from build123d import *

# Parameters (mm, degrees)
F1_DEPTH = 50.8
F3_DEPTH = 25.4
F4_W     = 12.7
F4_H     = 20.7277986608
F5_DEPTH = 19.05
F7_DEPTH = 25.4


with BuildPart() as f1:
    # F0 (on Right) → F1 (new body)
    with BuildSketch(Plane.YZ):
        Polygon((0, 0), (0, 31.7254364491), (-12.6999762453, 31.75), (-12.6999762453, 12.7), (-33.4277749062, 12.7), (-33.4277749062, 0), align=None)
    extrude(amount=F1_DEPTH)

    # F2 (on face) → F3 (cut)
    with BuildSketch(Plane.XZ.offset(12.6999762453)):
        Polygon((50.8, 31.75), (35.5220995843, 31.75), (50.8, 12.7), align=None)
    extrude(amount=-F3_DEPTH, mode=Mode.SUBTRACT)

    # F4 (on face) → F5 (join)
    with BuildSketch(Plane.XY.offset(12.7)):
        with Locations((25.4, -23.0638755757)):
            Rectangle(F4_W, F4_H)
    extrude(amount=F5_DEPTH)

    # F6 (on face) → F7 (cut)
    with BuildSketch(Plane.YZ.offset(31.75)):
        Polygon((-33.4277749062, 31.75), (-33.4277749062, 12.7), (-12.6999762453, 31.75), align=None)
    extrude(amount=-F7_DEPTH, mode=Mode.SUBTRACT)


solid = f1.part
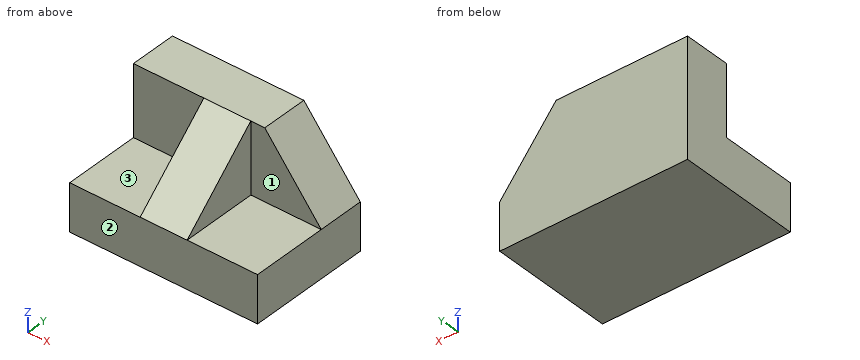
Could you check a few things on this model? Use its own coordinates, in mm. Face numbers are marked on the shaded views. A direction names the side the tool comes from. Round coordinates to 2 decimals unless told otherwise and drop trailing zeros. Loops run counter-clockwise (first coordinate to the right, second up) from the corner with the lowest first, then second, coordinate; pieces in that order, holes last. Notation, with made-up numbers: (86, 67.25) - (99, 67.25) arc R26 cw to (99, 94.25) - close; hole circle Ø2 at (25, 22.25). An arc over 180 degrees is marked (long way). Write item = value, one per line.
1) I'm going to push flat-ended pins straight in: P1, Ø15, axis at x = 38.5, y = -27, coming from the +Z side; P2, Ø5.5, axis at y = -18.5, z = 26.5, coming from the +X side; P3, Ø9.5, axis at y = -21, z = 25.5, coming from the -X side. Where does each tip first touch, or does it pass through?
Computed:
P1 = 21.61
P2 = 31.75
P3 = 19.05
2) Imagine slicing it at B-B (z = 17). Please give me the cut outline in (x, y).
Computed:
outline = (0, -12.7) - (19.05, -12.7) - (19.05, -28.75) - (31.75, -28.75) - (31.75, -12.7) - (47.35, -12.7) - (47.35, 0) - (0, 0) - close
3) Imagine slicing it at C-C (y = -15). Please give me the cut outline in (x, z), and give its area (3 significant figures).
Computed:
outline = (0, 0) - (50.8, 0) - (50.8, 12.7) - (31.75, 12.7) - (31.75, 29.64) - (19.05, 29.64) - (19.05, 12.7) - (0, 12.7) - close
area = 860 mm2
4) Imagine slicing it at A-A (x = 4). Please give me the cut outline in (y, z).
Computed:
outline = (-33.43, 0) - (0, 0) - (0, 31.73) - (-12.7, 31.75) - (-12.7, 12.7) - (-33.43, 12.7) - close
5) Imagine slicing it at D-D (x = 26.5). Please give me the cut outline in (y, z), and give its area (3 significant figures).
Computed:
outline = (-33.43, 0) - (0, 0) - (0, 31.73) - (-12.7, 31.75) - (-33.43, 12.7) - close
area = 864 mm2
6) I need wall thicknesses on line 1 along Z through (x, y) = (3, -1.5); line 2 along Y through (x, z) = (18, 28); line 3 along Z through (x, y) = (17.5, -23.5). Which ranges of each line are inside material? Lowest first, please. Write a range as from..to.
Computed:
line_1 = 0..31.73
line_2 = -12.7..0
line_3 = 0..12.7
7) On a 3-axis mill with a long thin cutter (end or side, diameter ignored), from which of +Z, -Z, +X, -X, +Y, -Y can I reach the whole of each face in a straight line? I mean the marked faces 1, 2 and 3. Say none if no direction works.
Computed:
face_1 = +Z, +X, -Y
face_2 = +Z, -Z, +X, -X, -Y
face_3 = +Z, -X, -Y
